Here's how the part is built. I have some questions about the finished solid (model axes, mm). A direction names the side the tool comes from. Round coordinates to 2 decimals unless told otherwise and drop trailing zeros. Write each loop counter-clockwise with the first axis right and the second up, starting at its lowest first coordinate (ties: lowest second). Pieces come first, ordered by that corner, then holes. Notation, with made-up numbers: M 78,79.5 L 94,79.5 A12 ccw 94,95.5 Z; hole C 33.5,84 d2. An arc over 180 degrees is marked long. Write item = value, one per line. Start each with the question number.
(1) I need wall thicknesses on line 1 along X through (y, z) = (6.75, 22.5); line 2 along Y through (x, z) = (333.5, -14). Which ranges of each line are inside material? Lowest first, please.
(2) I want a section at A-A (z = 10.5). List the corners of the cut face in (x, y) for me (3 decimals).
(3) Will these pins go through, and if not, where does the flat tip stop? pin 1 Ø11.5 at (x, z) = (343, -15.5) entering from -Y; pin 2 Ø4 at (x, y) = (-355, 2) entering from +Z (3 decimals).
(4) On a 3-axis mill with a long thin cutter (end or side, diameter ignored), from which of +Z, -Z, +X, -X, +Y, -Y can I reach the whole of each face in a straight line? I mean faces 1 (the flat face through (349, 0, 34.925)), 2 (the flat face through (-349, 0, -34.925)), 3 (the flat face through (-349, -6.35, 0)), 4 (the flat face through (-349, 0, 34.925)). Say none if no direction works.
```python
from build123d import *

# Parameters (mm, degrees)
F0_W     = 660.4
F0_H     = 76.2
F1_DEPTH = 9.525
F2_W     = 12.7
F2_H     = 69.85
F3_W     = 12.7
F3_H     = 69.85
F4_DEPTH = 38.1
F5_DEPTH = 38.1


with BuildPart() as f1:
    # F0 (on Front) → F1 (new body, symmetric)
    with BuildSketch(Plane.XZ):
        Rectangle(F0_W, F0_H)
    extrude(amount=F1_DEPTH, both=True)

    # F2 (on face) + F3 (on face) → F4 (join)
    with BuildSketch(Plane.YZ.offset(330.2)):
        Rectangle(F2_W, F2_H)
    with BuildSketch(Plane(origin=(-330.2, 0, 0), x_dir=(0, -1, 0), z_dir=(-1, 0, 0))):
        Rectangle(F3_W, F3_H)
    extrude(amount=F4_DEPTH)

    # F3 (on face) → F5 (join)
    with BuildSketch(Plane(origin=(-330.2, 0, 0), x_dir=(0, -1, 0), z_dir=(-1, 0, 0))):
        Rectangle(F3_W, F3_H)
    extrude(amount=F5_DEPTH)


solid = f1.part
```
Returned:
q1.line_1 = -330.2 to 330.2
q1.line_2 = -6.35 to 6.35
q2.outline = M -368.3,-6.35 L -330.2,-6.35 L -330.2,-9.525 L 330.2,-9.525 L 330.2,-6.35 L 368.3,-6.35 L 368.3,6.35 L 330.2,6.35 L 330.2,9.525 L -330.2,9.525 L -330.2,6.35 L -368.3,6.35 Z
q3.pin_1 = -6.35
q3.pin_2 = 34.925
q4.face_1 = +Z, +X, +Y, -Y
q4.face_2 = -Z, -X, +Y, -Y
q4.face_3 = +Z, -Z, -X, -Y
q4.face_4 = +Z, -X, +Y, -Y
